from build123d import *

# Parameters (mm, degrees)
SKETCH1_R           = 16
SKETCH1_R_2         = 9
SKETCH1_R_3         = 1.95
SKETCH1_R_4         = 7
BOSS_EXTRUDE1_DEPTH = 2
SKETCH1_3_R         = 9
SKETCH1_3_R_2       = 7
BOSS_EXTRUDE2_DEPTH = 13
SKETCH2_R           = 2
CUT_EXTRUDE1_DEPTH  = 13


with BuildPart() as part:
    # Sketch1 → Boss-Extrude1 (new body)
    # profile 1 of 2: a face of its own
    with BuildSketch(Plane(origin=(0, 0, 0), x_dir=(0, 1, 0), z_dir=(0, 0, 1))):
        with Locations(Location((0, 0, 0), (0, 0, 270))):
            Circle(SKETCH1_R)
        Circle(SKETCH1_R_2, mode=Mode.SUBTRACT)
        with Locations(Location((9, 9, 0), (0, 0, 270))):
            Circle(SKETCH1_R_3, mode=Mode.SUBTRACT)
        with Locations(Location((9, -9, 0), (0, 0, 270))):
            Circle(SKETCH1_R_3, mode=Mode.SUBTRACT)
        with Locations(Location((-9, -9, 0), (0, 0, 270))):
            Circle(SKETCH1_R_3, mode=Mode.SUBTRACT)
        with Locations(Location((-9, 9, 0), (0, 0, 270))):
            Circle(SKETCH1_R_3, mode=Mode.SUBTRACT)
    # profile 2 of 2: a face of its own
    with BuildSketch(Plane(origin=(0, 0, 0), x_dir=(0, 1, 0), z_dir=(0, 0, 1))):
        Circle(SKETCH1_R_2)
        with Locations(Location((0, 0, 0), (0, 0, 270))):
            Circle(SKETCH1_R_4, mode=Mode.SUBTRACT)
    extrude(amount=BOSS_EXTRUDE1_DEPTH)

    # Sketch1_3 → Boss-Extrude2 (add)
    with BuildSketch(Plane(origin=(0, 0, 0), x_dir=(0, 1, 0), z_dir=(0, 0, 1))):
        with Locations(Location((0, 0, 0), (0, 0, 90))):
            Circle(SKETCH1_3_R)
        with Locations(Location((0, 0, 0), (0, 0, 270))):
            Circle(SKETCH1_3_R_2, mode=Mode.SUBTRACT)
    extrude(amount=BOSS_EXTRUDE2_DEPTH)

    # Sketch2 → Cut-Extrude1 (cut)
    with BuildSketch(Plane(origin=(0, 0, 0), x_dir=(-1, 0, 0), z_dir=(0, 1, 0))):
        with Locations(Location((0, 8, 0), (0, 0, 90))):
            Circle(SKETCH2_R)
    extrude(amount=-CUT_EXTRUDE1_DEPTH, mode=Mode.SUBTRACT)


solid = part.part
Verification items for the finished model (mm, model axes). A direction names the side the tool comes from. Coordinates: 2 decimals unless noted, no trailing zeros. Order: outer loops, then holes, each group sorted by start corner. A loop starts at its lowest first (then second) coordinate and runs counter-clockwise, first axis right, second up. Notation, with made-up numbers: (39.25, 48) -> (93.25, 48) arc R29 ccw to (93.25, 81) -> close; hole circle Ø7 at (83.5, 23.5). An arc over 180 degrees is marked (long way). Use CSV: the item, a comma, the result in double quotes. Start each with the question number.
Q1. Section check B-B, the plane z = 1.5. Record the cut outline in (x, y), and give its area (3 significant figures).
Q2. Section check A-A, the plane x = 0. Record the cut outline in (y, z).
Q3. Section check C-C, the plane y = 10. Record the cut outline in (x, z), and give its area (3 significant figures).
Q4. Section check D-D, the plane x = -5. Record the cut outline in (y, z).
Q5. Tool access check on faces 1 (the flat face through (0, 7.3, 13)), 2 (the cylindrical face through (-1.2, -7.8, 6.4)), 3 (the cylindrical face through (1.951, 8.786, 7.423)). Record the directions out of +Z, -Z, +X, -X, +Y, -Y that give a thin tool (end or side, any length) a straight path to the whole face; none if there is none.
Q6. Depth check by flat-ended pin: P1, Ø6, axis at y = 2, z = 8.5, coming from the +X side; P2, Ø10, axis at x = 4, y = -11.5, coming from the -Z side; P3, Ø4, axis at x = -8, z = 11.5, coming from the +Y side; P4, Ø2, axis at x = 2, z = 2.5, coming from the -Y side. Enter the tip coordinate at first touch or a pass-through.
Q7. Draft check along X on faces 4 (the cylindrical face through (-7.952, 10.644, 0.986)), 5 (the cylindrical face through (-3.47, -15.62, 0.99)), 6 (the flat face through (7, 7, 2)), 7 (the cylindrical face through (3.763, 5.902, 6.409)). Enter one of: +X half, -X half, draft (parallel to the pull), parting line (faces both ways), or undercut.
Q8. Thickness scan on line 1 along Y through (x, z) = (0, 5.25); line 2 along Z through (x, y) = (6.5, -11.5); line 3 along X through (y, z) = (7.5, 0.75). Record the ranges inside material, lowest first.
Returned:
1,outline,"circle Ø32 at (0, 0); hole circle Ø3.9 at (-9, -9); hole circle Ø3.9 at (-9, 9); hole circle Ø14 at (0, 0); hole circle Ø3.9 at (9, -9); hole circle Ø3.9 at (9, 9)"
1,area,"603 mm^2"
2,outline,"(-16, 0) -> (-7, 0) -> (-7, 6) -> (-9, 6) -> (-9, 2) -> (-16, 2) -> close; (-9, 10) -> (-7, 10) -> (-7, 13) -> (-9, 13) -> close; (7, 0) -> (16, 0) -> (16, 2) -> (9, 2) -> (9, 13) -> (7, 13) -> close"
3,outline,"(-12.49, 0) -> (-10.67, 0) -> (-10.67, 2) -> (-12.49, 2) -> close; (-7.33, 0) -> (7.33, 0) -> (7.33, 2) -> (-7.33, 2) -> close; (10.67, 0) -> (12.49, 0) -> (12.49, 2) -> (10.67, 2) -> close"
3,area,"36.6 mm^2"
4,outline,"(-15.2, 0) -> (-4.9, 0) -> (-4.9, 13) -> (-7.48, 13) -> (-7.48, 2) -> (-15.2, 2) -> close; (4.9, 0) -> (15.2, 0) -> (15.2, 2) -> (7.48, 2) -> (7.48, 13) -> (4.9, 13) -> close"
5,face 1,"+Z, +X, -X, +Y, -Y"
5,face 2,"-Y"
5,face 3,"+Z"
6,P1,"stops at x = 9"
6,P2,"stops at z = 0"
6,P3,"stops at y = 6.71"
6,P4,"stops at y = -15.96"
7,face 4,"undercut"
7,face 5,"parting line"
7,face 6,"draft"
7,face 7,"undercut"
8,line 1,"y = -9 to -7, 7 to 9"
8,line 2,"z = 0 to 2"
8,line 3,"x = -14.13 to -10.25, -7.75 to 7.75, 10.25 to 14.13"
